Read the model definition and answer for the solid it produces. Units are mm, in the model's axes. Coordinates: 2 decimals unless noted, no trailing zeros. Write each loop counter-clockwise with the first axis right and the second up, starting at its lowest first coordinate (ties: lowest second). Pieces come first, ordered by that corner, then holes.
(1) Section A-A on y = 104.5 is taken. Write down the section's boundary in (x, z).
(2) Given pin 1 (1 mm diameter, centred on x = 0, z = 1, fed in from -Y); pin 2 (2 mm diameter, centred on x = 1, z = 2, fed in from -Y), each flat-ended and moving along its own axis, determine where each tip first touches the part or whether it passes through.
(3) Find the intervals of material crossed by probe 1 along X at (y, z) = (63, -3.25); probe 2 along X at (y, z) = (86.5, -1.25); probe 3 along Z at (x, y) = (3, 128.5), in increasing order.
(4) Section B-B on x = 0 is taken. Write down the section's boundary in (y, z), then the cut area to 3 significant figures.
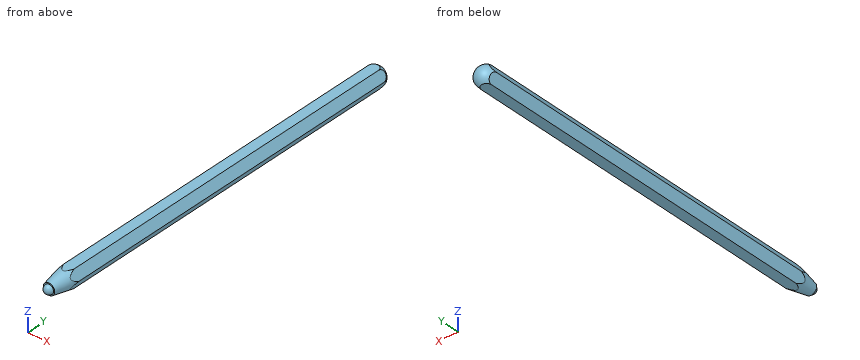
Autodesk Inventor part; units mm, degrees
ref_plane "YZ Plane" through (0, 0, 0) normal (1, 0, 0) x (0, 1, 0)
ref_plane "XZ Plane" through (0, 0, 0) normal (0, 1, 0) x (-1, 0, 0)
ref_plane "XY Plane" through (0, 0, 0) normal (0, 0, 1) x (1, 0, 0)
sketch "Sketch1" plane through (0, 0, 0) normal (0, 1, 0) x (-1, 0, 0)
  line L0 (-4.5, 0) -> (-2.25, 3.8971)
  line L1 (-2.25, 3.8971) -> (2.25, 3.8971)
  line L2 (2.25, 3.8971) -> (4.5, 0)
  line L3 (4.5, 0) -> (2.25, -3.8971)
  line L4 (2.25, -3.8971) -> (-2.25, -3.8971)
  line L5 (-2.25, -3.8971) -> (-4.5, 0)
  point P0 (0, 0)
  point P1 (0, 0)
  dimension "d1" = 9
extrude "Extrusion1" add sketch "Sketch1" along normal blind 155
sketch "Sketch2" plane through (0, 0, 0) normal (0, 0, 1) x (1, 0, 0)
  line L0 (2.25, 155) -> (-2.25, 155)
  line L1 (2.25, 155) -> (4.5, 155)
  arc A0 (4.5, 155) -> (0, 159.5) centre (0, 155) ccw
  line L2 (0, 155) -> (0, 159.5)
  line L3 (0, 155) -> (4.5, 155)
  point P0 (0, 0)
revolve "Revolution1" add sketch "Sketch2" angle 360 about axis through (0, 155, 0) along (0, 1, 0)
sketch "Sketch3" plane through (0, 0, 0) normal (0, -1, 0) x (1, 0, 0)
  line L0 (2.25, -3.8971) -> (-2.25, -3.8971)
  arc A0 (-4.5, 0) -> (-2.25, -3.8971) centre (0, 0) ccw
  line L1 (2.25, -3.8971) -> (-2.25, -3.8971)
  line L2 (-2.25, -3.8971) -> (-4.5, 0)
  line L3 (-2.25, -3.8971) -> (-4.5, 0)
  arc A1 (-2.25, 3.8971) -> (-4.5, 0) centre (0, 0) ccw
  line L4 (-4.5, 0) -> (-2.25, 3.8971)
  arc A2 (2.25, 3.8971) -> (-2.25, 3.8971) centre (0, 0) ccw
  line L5 (-2.25, 3.8971) -> (2.25, 3.8971)
  line L6 (2.25, 3.8971) -> (4.5, 0)
  line L7 (4.5, 0) -> (2.25, -3.8971)
  point P0 (0, 0)
extrude "Extrusion2" cut sketch "Sketch3" along normal mid plane 400 contours L0 L2 L4 L5 L6 L7 keep common part
sketch "Sketch4" plane through (0, 0, 0) normal (0, 0, 1) x (1, 0, 0)
  line L0 (-4.5, 0) -> (-4.5, 155)
  line L1 (0, 0) -> (-4.5, 0)
  line L2 (0, 0) -> (0, -10)
  line L3 (0, -10) -> (-2.5, -10)
  line L4 (-4.5, 0) -> (-2.5, -10)
  point P0 (-4.5, 100)
  dimension "d7" = 10
  dimension "d9" = 2.5
revolve "Revolution2" add sketch "Sketch4" angle 360 about axis through (0, 0, 0) along (0, -1, 0)
thicken "Thicken1" operation cut thickness 5 both sides no extend neighbours no toward (0, -1, 0) faces at (-0.4635, 0, 4.0247)
thicken "Thicken2" operation cut thickness 5 both sides no extend neighbours no toward (0, -1, 0) faces at (-3.2537, 0, 2.4138)
thicken "Thicken3" operation cut thickness 5 both sides no extend neighbours no toward (0, -1, 0) faces at (-3.7172, 0, -1.6109)
thicken "Thicken4" operation cut thickness 5 both sides no extend neighbours no toward (0, -1, 0) faces at (3.4635, 0, 2.1807)
thicken "Thicken5" operation cut thickness 5 both sides no extend neighbours no toward (0, -1, 0) faces at (3.7172, 0, -1.6109)
thicken "Thicken6" operation cut thickness 5 both sides no extend neighbours no toward (0, -1, 0) faces at (0.1568, 0, -4.0899)
sketch "Sketch5" plane through (0, 0, 0) normal (0, 0, 1) x (1, 0, 0)
  line L0 (-2.5, -10) -> (2.5, -10)
  arc A0 (2, -10) -> (0, -12) centre (0, -10) ccw
  line L1 (0, -10) -> (0, -12)
  line L2 (2.5, -10) -> (2, -10)
  line L3 (-2, -10) -> (-2.5, -10)
  line L4 (0, -10) -> (-2, -10)
  point P0 (0, 0)
  point P1 (-2, -10)
  dimension "d23" = 4
revolve "Revolution3" add sketch "Sketch5" angle 360 about axis through (0, -10, 0) along (0, -1, 0) contours L0 L1 A0
properties part number "stylus_pen" material "Acetal Resin, White"
Response:
1. outline: (-4.5, 0) - (-2.25, -3.9) - (2.25, -3.9) - (4.5, 0) - (2.25, 3.9) - (-2.25, 3.9) - close
2. pin 1: stops at y = -11.94
2. pin 2: stops at y = -11.57
3. probe 1: x = -2.62 to 2.62
3. probe 2: x = -3.78 to 3.78
3. probe 3: z = -2.6 to 2.6
4. outline: (-10, -2.5) - (-3.01, -3.9) - (157.25, -3.9) arc R4.5 ccw to (157.25, 3.9) - (-3.01, 3.9) - (-10, 2.5) - (-10, 2) arc R2 ccw to (-10, -2) - close
4. area: 1,310 mm2
